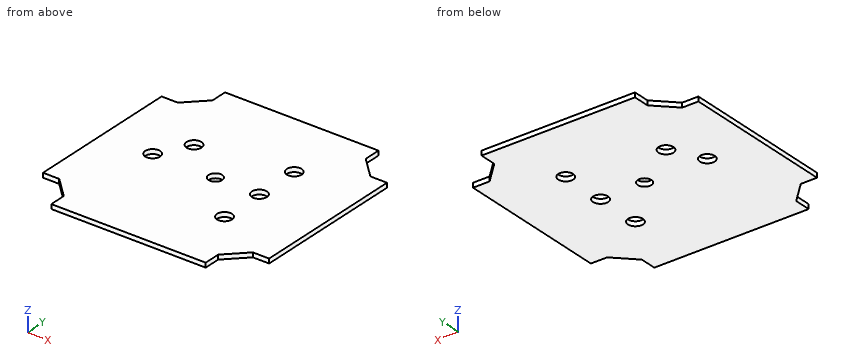
Autodesk Inventor part; units mm, degrees
ref_plane "Work Plane1" through (-29.1, -14.5, 2.4) normal (0, 0, -1) x (0, 1, 0)
ref_plane "Work Plane2" through (-13.8999, -10.5497, 2.25) normal (0, 0, -1) x (0, 1, 0)
ref_plane "YZ Plane" through (0, 0, 0) normal (1, 0, 0) x (0, 1, 0)
ref_plane "Work Plane1" through (-29.1, -14.5, 2.4) normal (0, 0, -1) x (0, 1, 0)
ref_plane "Work Plane2" through (-13.8999, -10.5497, 2.25) normal (0, 0, -1) x (0, 1, 0)
sketch "Sketch1" plane through (0, 0, 0) normal (0, 0, 1) x (1, 0, 0)
  line L0 (-34.86, 0) -> (34.86, 0) construction
  line L1 (0, -34.86) -> (0, 34.86) construction
  line L2 (0, 0) -> (11.1575, 11.1575) construction
  line L3 (0, 0) -> (15.7791, 0) construction
  line L4 (0, 24.9) -> (16.8009, 24.9)
  line L5 (16.8009, 24.9) -> (16.8009, 21.2415)
  line L6 (16.8009, 21.2415) -> (19.0212, 19.0212)
  line L7 (24.9, 0) -> (24.9, 16.8009)
  line L8 (24.9, 16.8009) -> (21.2415, 16.8009)
  line L9 (21.2415, 16.8009) -> (19.0212, 19.0212)
  line L10 (0, -24.9) -> (16.8009, -24.9)
  line L11 (16.8009, -24.9) -> (16.8009, -21.2415)
  line L12 (16.8009, -21.2415) -> (19.0212, -19.0212)
  line L13 (24.9, 0) -> (24.9, -16.8009)
  line L14 (24.9, -16.8009) -> (21.2415, -16.8009)
  line L15 (21.2415, -16.8009) -> (19.0212, -19.0212)
  line L16 (0, 24.9) -> (-16.8009, 24.9)
  line L17 (-16.8009, 24.9) -> (-16.8009, 21.2415)
  line L18 (-16.8009, 21.2415) -> (-19.0212, 19.0212)
  line L19 (-24.9, 16.8009) -> (-21.2415, 16.8009)
  line L20 (-21.2415, 16.8009) -> (-19.0212, 19.0212)
  line L21 (0, -24.9) -> (-16.8009, -24.9)
  line L22 (-16.8009, -24.9) -> (-16.8009, -21.2415)
  line L23 (-16.8009, -21.2415) -> (-19.0212, -19.0212)
  line L24 (-21.2415, -16.8009) -> (-19.0212, -19.0212)
  line L25 (-24.9, -16.8009) -> (-21.2415, -16.8009)
  line L26 (-24.9, 0) -> (-24.9, -16.8009)
  line L27 (-24.9, 0) -> (-24.9, 16.8009)
  circle A0 centre (0, 0) radius 1.5
  dimension "d0" = 45
  dimension "d2" = 24.9
  dimension "d3" = 3.14
  dimension "d4" = 26.9
  dimension "d5" = 3
extrude "Extrusion1" add sketch "Sketch1" along normal blind 1
sketch "Sketch5" plane through (0, 0, 0) normal (0, 0, -1) x (-1, 0, 0)
  circle A0 centre (-9.7, 10) radius 1.4
  circle A1 centre (-9.7, -10) radius 1.4
  circle A2 centre (13.8, 0) radius 1.4
  circle A3 centre (-10, 6.9) radius 0.75
  circle A4 centre (10, 6.9) radius 1.25
  circle A5 centre (-9.7, 0) radius 1.5
  point P0 (0, 0)
  dimension "d28" = 3
hole "Hole1" at (-13.8, 0, 0) at (9.7, -10, 0) at (-10, 6.9, 0) at (9.7, 10, 0) at (9.7, 0, 0) direction (0, 0, 1) diameter 3.3 depth 12 tip angle 118
sketch "Skizze6" plane through (-16.8009, 24.9, 1) normal (0, 0, 1) x (1, 0, 0)
  circle A0 centre (6.8009, -18) radius 1.65 construction
  circle A1 centre (3.0009, -24.9) radius 1.65 construction
  circle A2 centre (26.5009, -34.9) radius 1.65 construction
  circle A3 centre (26.5009, -14.9) radius 1.65 construction
  circle A4 centre (16.8009, -24.9) radius 10 construction
  line L0 (33.6017, -3.6585) -> (33.6017, 0)
  line L1 (33.6017, 0) -> (0, 0) construction
  line L2 (0, 0) -> (0, -3.6585)
  line L3 (0, -3.6585) -> (-4.4406, -8.0991)
  line L4 (-4.4406, -8.0991) -> (-8.0991, -8.0991)
  line L5 (-8.0991, -8.0991) -> (-8.0991, -41.7009) construction
  line L6 (-8.0991, -41.7009) -> (-4.4406, -41.7009)
  line L7 (-4.4406, -41.7009) -> (0, -46.1415)
  line L8 (0, -46.1415) -> (0, -49.8)
  line L9 (0, -49.8) -> (33.6017, -49.8) construction
  line L10 (33.6017, -49.8) -> (33.6017, -46.1415)
  line L11 (33.6017, -46.1415) -> (38.0423, -41.7009)
  line L12 (38.0423, -41.7009) -> (41.7009, -41.7009)
  line L13 (41.7009, -41.7009) -> (41.7009, -8.0991) construction
  line L14 (41.7009, -8.0991) -> (38.0423, -8.0991)
  line L15 (38.0423, -8.0991) -> (33.6017, -3.6585)
  line L16 (-0.2, 0.2) -> (33.8017, 0.2) construction
  line L17 (33.8017, 0.2) -> (33.8017, -3.5757)
  line L18 (33.8017, -3.5757) -> (38.1252, -7.8991)
  line L19 (38.1252, -7.8991) -> (41.9009, -7.8991)
  line L20 (41.9009, -7.8991) -> (41.9009, -41.9009) construction
  line L21 (41.9009, -41.9009) -> (38.1252, -41.9009)
  line L22 (38.1252, -41.9009) -> (33.8017, -46.2243)
  line L23 (33.8017, -46.2243) -> (33.8017, -50)
  line L24 (33.8017, -50) -> (-0.2, -50) construction
  line L25 (-0.2, -50) -> (-0.2, -46.2243)
  line L26 (-0.2, -46.2243) -> (-4.5235, -41.9009)
  line L27 (-4.5235, -41.9009) -> (-8.2991, -41.9009)
  line L28 (-8.2991, -41.9009) -> (-8.2991, -7.8991) construction
  line L29 (-8.2991, -7.8991) -> (-4.5235, -7.8991)
  line L30 (-4.5235, -7.8991) -> (-0.2, -3.5757)
  line L31 (-0.2, -3.5757) -> (-0.2, 0.2)
  line L32 (-8.0991, -8.0991) -> (-8.0991, -7.8991)
  line L33 (0, 0) -> (-0.2, 0)
  line L34 (33.6017, 0) -> (33.8017, 0)
  line L35 (41.7009, -8.0991) -> (38.0423, -8.0991)
  line L36 (41.7009, -8.0991) -> (41.7009, -7.8991)
  line L37 (41.7009, -41.7009) -> (41.7009, -41.9009)
  line L38 (33.6017, -49.8) -> (33.8017, -49.8)
  line L39 (-8.0991, -41.7009) -> (-8.0991, -41.9009)
  line L40 (0, -49.8) -> (-0.2, -49.8)
  point P0 (16.8009, -24.9)
  dimension "d25" = 0.2
extrude "IM_offset" add sketch "Skizze6" against normal up to surface (1 mm away) contours L2 L3 L4 L32 L29 L30 L31 L33 | L6 L7 L8 L40 L25 L26 L27 L39 | L10 L11 L12 L37 L21 L22 L23 L38
properties part number "20_Cube_insert_AlliedVision_Alvium_v3"
Geometry: final body of the model. Coordinates: model frame, mm. Give positions to 0.01 mm unless a question says otherwise; leave off trailing zeros. Write each loop counter-clockwise with the first axis right and the second up, starting at its lowest first coordinate (ties: lowest second). Pieces come first, ordered by that corner, then holes. Notation, with made-up numbers: (38.25, 10.5) - (48.25, 10.5) arc R7 cw to (48.25, 23.5) - close; hole circle Ø1 at (-12.75, -5). An arc over 180 degrees is marked (long way). Return JSON: item names as keys, results as strings. Group by question number.
1) Section C-C on y = -10. Return the cut outline in (x, z), plus the area to 3 significant figures.
2) Section B-B on x = -13.8. Return the cut outline in (y, z).
3) Section A-A on y = 0. Return the cut outline in (x, z).
4) First-contact query: P1, Ø0.5, axis at x = -22.5, z = 0.5, coming from the -Y side; P2, Ø0.5, axis at y = 23, z = 0.5, coming from the -X side; P3, Ø0.5, axis at x = -23, z = 0.5, coming from the +Y side. Flat tips, straight axial feed; report the tip coordinate or a pass-through.
5) Section D-D on z = 0.2. Return the cut outline in (x, y), plus the area to 3 significant figures.
6) Line query: line 1 (Y direction, x = 9.7, z = 0.7); line 2 (X direction, y = 6.9, z = 0.5); line 3 (X direction, y = 7.5, z = 0.8). Output: solid intervals per line, ascending.
Filled in:
{
 "1": {"outline": "(-24.9, 0) - (8.05, 0) - (8.05, 1) - (-24.9, 1) - close; (11.35, 0) - (24.9, 0) - (24.9, 1) - (11.35, 1) - close", "area": "46.5 mm^2"},
 "2": {"outline": "(-24.9, 0) - (-1.65, 0) - (-1.65, 1) - (-24.9, 1) - close; (1.65, 0) - (24.9, 0) - (24.9, 1) - (1.65, 1) - close"},
 "3": {"outline": "(-24.9, 0) - (-15.45, 0) - (-15.45, 1) - (-24.9, 1) - close; (-12.15, 0) - (-1.5, 0) - (-1.5, 1) - (-12.15, 1) - close; (1.5, 0) - (8.05, 0) - (8.05, 1) - (1.5, 1) - close; (11.35, 0) - (24.9, 0) - (24.9, 1) - (11.35, 1) - close"},
 "4": {"P1": "stops at y = -17", "P2": "stops at x = -17", "P3": "stops at y = 17"},
 "5": {"outline": "(-24.9, -17) - (-21.32, -17) - (-17, -21.32) - (-17, -24.9) - (17, -24.9) - (17, -21.32) - (21.32, -17) - (24.9, -17) - (24.9, 16.8) - (21.24, 16.8) - (16.8, 21.24) - (16.8, 24.9) - (-17, 24.9) - (-17, 21.32) - (-21.32, 17) - (-24.9, 17) - close; hole circle Ø3.3 at (-13.8, 0); hole circle Ø3.3 at (-10, 6.9); hole circle Ø3 at (0, 0); hole circle Ø3.3 at (9.7, -10); hole circle Ø3.3 at (9.7, 0); hole circle Ø3.3 at (9.7, 10)", "area": "2,220 mm^2"},
 "6": {"line 1": "y = -24.9 to -11.65, -8.35 to -1.65, 1.65 to 8.35, 11.65 to 24.9", "line 2": "x = -24.9 to -11.65, -8.35 to 24.9", "line 3": "x = -24.9 to -11.54, -8.46 to 24.9"}
}
